Could you check a few things on this model? Use its own coordinates, in mm. Face numbers are marked on the shaded views. A direction names the side the tool comes from. Give positions to 0.01 mm unless a question says otherwise; leave off trailing zeros. Order: outer loops, then holes, each group sorted by start corner. A loop starts at its lowest first (then second) coordinate and runs counter-clockwise, first axis right, second up. Notation, with made-up numbers: (36.5, 69) - (69.5, 69) arc R11 cw to (69.5, 79) - close; hole circle Ø9 at (22.25, 80). An arc over 180 degrees is marked (long way). One line per question, with ' | ' between items. Start each with the question number.
1. Imagine slicing it at A-A (y = 31). Please give me the cut outline in (x, z).
2. Imagine slicing it at B-B (x = 5.5). Please give me the cut outline in (y, z), and give its area (4 significant figures).
3. Which directions (+Z, -Z, +X, -X, +Y, -Y) give clear straight access to the entire face, cutting with the end or side of a thin tool? Please do the marked faces 1 and 2.
4. For P1, Ø15, axis at x = 4, y = 34, coming from the -Z side, with a flat end and sliding along its axis, tell me the tip position at first contact or that it passes through.
5. I need wall thicknesses on probe 1 along Z at (x, y) = (-3, 23); probe 2 along Y at (x, z) = (-14, -2); probe 3 along X at (y, z) = (45, 0.5). Which ranges of each line are inside material? Lowest first, please. Write a range as from..to.
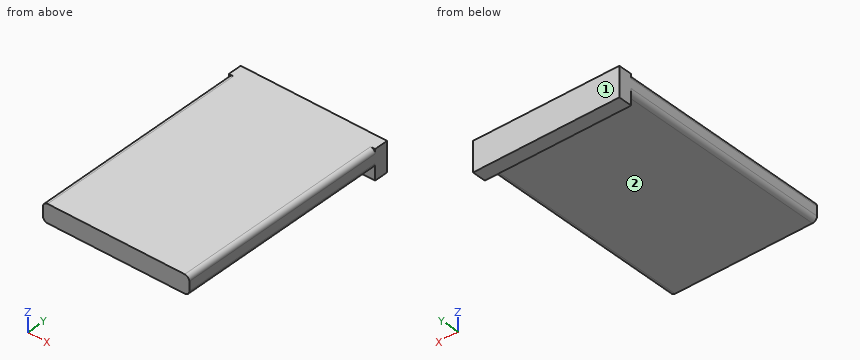
```python
from build123d import *

# Parameters (mm, degrees)
SKETCH1_W      = 32
SKETCH1_H      = 50
EXTRUDE1_DEPTH = 4
FILLET1_R      = 1
SKETCH3_W      = 32
SKETCH3_H      = 6.5
EXTRUDE3_DEPTH = 3


with BuildPart() as part:
    # Sketch1 → Extrude1 (new body)
    with BuildSketch(Plane.XY):
        with Locations((0, 25)):
            Rectangle(SKETCH1_W, SKETCH1_H)
    extrude(amount=EXTRUDE1_DEPTH)

    # Fillet1
    fillet1_edges = [part.edges().sort_by_distance(p)[0] for p in [
        (16, 25, 4),
        (-16, 25, 4),
        (16, 25, 0),
        (-16, 25, 0),
    ]]
    fillet(fillet1_edges, radius=FILLET1_R)

    # Sketch3 → Extrude3 (add)
    with BuildSketch(Plane(origin=(0, 50, 0), x_dir=(1, 0, 0), z_dir=(0, 1, 0))):
        with Locations((0, -0.75)):
            Rectangle(SKETCH3_W, SKETCH3_H)
    extrude(amount=-EXTRUDE3_DEPTH)


solid = part.part
```
Results found:
1) outline: (-16, 1) arc R1 ccw to (-15, 0) - (15, 0) arc R1 ccw to (16, 1) - (16, 3) arc R1 ccw to (15, 4) - (-15, 4) arc R1 ccw to (-16, 3) - close
2) outline: (0, 0) - (47, 0) - (47, -2.5) - (50, -2.5) - (50, 4) - (0, 4) - close | area: 207.5 mm2
3) face 1: +Z, -Z, +X, -X, +Y | face 2: -Z, +X, -X, -Y
4) P1: stops at z = 0
5) probe 1: z = 0..4 | probe 2: y = 47..50 | probe 3: x = -15.87..15.87
